The listing builds one solid part. Answer for the finished solid, in the listing's coordinates (mm). Give positions to 0.01 mm unless a question says otherwise; leave off trailing zeros. Write each loop counter-clockwise with the first axis right and the second up, starting at its lowest first coordinate (ties: lowest second). Pieces come first, ordered by that corner, then holes.
```python
from build123d import *
from build123d.topology import SkipClean

# Parameters (mm, degrees)
SKETCH1_R           = 31
SKETCH1_R_2         = 1.55
BOSS_EXTRUDE1_DEPTH = 2
BOSS_EXTRUDE2_START = 2
SKETCH3_R           = 11
BOSS_EXTRUDE2_DEPTH = 2
SKETCH4_R           = 4.5
CUT_EXTRUDE2_DEPTH  = 4
SKETCH2_R           = 8.2
CUT_EXTRUDE1_DEPTH  = 2


with BuildPart() as part:
    # Sketch1 → Boss-Extrude1 (new body)
    with BuildSketch(Plane.XY):
        Circle(SKETCH1_R)
        with Locations((-27, 0)):
            Circle(SKETCH1_R_2, mode=Mode.SUBTRACT)
        with Locations((-19.091883092, 19.091883092)):
            Circle(SKETCH1_R_2, mode=Mode.SUBTRACT)
        with Locations((0, 27)):
            Circle(SKETCH1_R_2, mode=Mode.SUBTRACT)
        with Locations((19.091883092, 19.091883092)):
            Circle(SKETCH1_R_2, mode=Mode.SUBTRACT)
        with Locations((27, 0)):
            Circle(SKETCH1_R_2, mode=Mode.SUBTRACT)
        with Locations((19.091883092, -19.091883092)):
            Circle(SKETCH1_R_2, mode=Mode.SUBTRACT)
        with Locations((0, -27)):
            Circle(SKETCH1_R_2, mode=Mode.SUBTRACT)
        with Locations((-19.091883092, -19.091883092)):
            Circle(SKETCH1_R_2, mode=Mode.SUBTRACT)
        with BuildLine():
            Line((-10.712142643, 2.5), (-22.86372673, 2.5))
            ThreePointArc((-22.86372673, 2.5), (-21.249229248, 8.801718944), (-17.934863167, 14.399329261))
            Line((-17.934863167, 14.399329261), (-9.342395657, 5.806861751))
            ThreePointArc((-9.342395657, 5.806861751), (-10.162674858, 4.209517756), (-10.712142643, 2.5))
        make_face(mode=Mode.SUBTRACT)
        with BuildLine():
            Line((-10.712142643, -2.5), (-22.86372673, -2.5))
            ThreePointArc((-22.86372673, -2.5), (-21.249229248, -8.801718944), (-17.934863167, -14.399329261))
            Line((-17.934863167, -14.399329261), (-9.342395657, -5.806861751))
            ThreePointArc((-9.342395657, -5.806861751), (-10.162674858, -4.209517756), (-10.712142643, -2.5))
        make_face(mode=Mode.SUBTRACT)
        with BuildLine():
            Line((-5.806861751, 9.342395657), (-14.399329261, 17.934863167))
            ThreePointArc((-14.399329261, 17.934863167), (-8.801718944, 21.249229248), (-2.5, 22.86372673))
            Line((-2.5, 22.86372673), (-2.5, 10.712142643))
            ThreePointArc((-2.5, 10.712142643), (-4.209517756, 10.162674858), (-5.806861751, 9.342395657))
        make_face(mode=Mode.SUBTRACT)
        with BuildLine():
            Line((2.5, 10.712142643), (2.5, 22.86372673))
            ThreePointArc((2.5, 22.86372673), (8.801718944, 21.249229248), (14.399329261, 17.934863167))
            Line((14.399329261, 17.934863167), (5.806861751, 9.342395657))
            ThreePointArc((5.806861751, 9.342395657), (4.209517756, 10.162674858), (2.5, 10.712142643))
        make_face(mode=Mode.SUBTRACT)
        with BuildLine():
            Line((9.342395657, 5.806861751), (17.934863167, 14.399329261))
            ThreePointArc((17.934863167, 14.399329261), (21.249229248, 8.801718944), (22.86372673, 2.5))
            Line((22.86372673, 2.5), (10.712142643, 2.5))
            ThreePointArc((10.712142643, 2.5), (10.162674858, 4.209517756), (9.342395657, 5.806861751))
        make_face(mode=Mode.SUBTRACT)
        with BuildLine():
            Line((10.712142643, -2.5), (22.86372673, -2.5))
            ThreePointArc((22.86372673, -2.5), (21.249229248, -8.801718944), (17.934863167, -14.399329261))
            Line((17.934863167, -14.399329261), (9.342395657, -5.806861751))
            ThreePointArc((9.342395657, -5.806861751), (10.162674858, -4.209517756), (10.712142643, -2.5))
        make_face(mode=Mode.SUBTRACT)
        with BuildLine():
            Line((5.806861751, -9.342395657), (14.399329261, -17.934863167))
            ThreePointArc((14.399329261, -17.934863167), (8.801718944, -21.249229248), (2.5, -22.86372673))
            Line((2.5, -22.86372673), (2.5, -10.712142643))
            ThreePointArc((2.5, -10.712142643), (4.209517756, -10.162674858), (5.806861751, -9.342395657))
        make_face(mode=Mode.SUBTRACT)
        with BuildLine():
            Line((-2.5, -10.712142643), (-2.5, -22.86372673))
            ThreePointArc((-2.5, -22.86372673), (-8.801718944, -21.249229248), (-14.399329261, -17.934863167))
            Line((-14.399329261, -17.934863167), (-5.806861751, -9.342395657))
            ThreePointArc((-5.806861751, -9.342395657), (-4.209517756, -10.162674858), (-2.5, -10.712142643))
        make_face(mode=Mode.SUBTRACT)
    extrude(amount=BOSS_EXTRUDE1_DEPTH)

    # Sketch3 → Boss-Extrude2 (add)
    with SkipClean():  # the faces are left unmerged after this step: merging them gives an invalid solid
        with BuildSketch(Plane(origin=(0, 0, 0), x_dir=(-1, 0, 0), z_dir=(0, 0, -1)).offset(BOSS_EXTRUDE2_START)):
            Circle(SKETCH3_R)
        extrude(amount=-BOSS_EXTRUDE2_DEPTH)

    # Sketch4 → Cut-Extrude2 (cut)
    with SkipClean():  # the faces are left unmerged after this step: merging them gives an invalid solid
        with BuildSketch(Plane.XY.offset(2)):
            Circle(SKETCH4_R)
        extrude(amount=-CUT_EXTRUDE2_DEPTH, mode=Mode.SUBTRACT)

    # Sketch2 → Cut-Extrude1 (cut)
    with SkipClean():  # the faces are left unmerged after this step: merging them gives an invalid solid
        with BuildSketch(Plane.XY.offset(2)):
            Circle(SKETCH2_R)
        extrude(amount=-CUT_EXTRUDE1_DEPTH, mode=Mode.SUBTRACT)


solid = part.part
```
Item 1: Each of these flat-tipped pins is pushed along its axis until it touches: P1, Ø3.5, axis at x = 19.09, y = -19.09, coming from the -Z side; P2, Ø1, axis at x = -16.5, z = 1.5, coming from the +Y side; P3, Ø2, axis at x = -15, z = 1, coming from the -Y side. Where does it stop, or does it pass through?
Conclusion:
P1: stops at z = 0
P2: stops at y = 26.55
P3: stops at y = -27.66
Item 2: Consider probe 1 along Y at (x, z) = (0, 0.05); probe 2 along Y at (x, z) = (-21, 1.7); probe 3 along Y at (x, z) = (5, 1.15). Determine where each line is inside the solid, lowest interval first.
Conclusion:
probe 1: y = -31 to -28.55, -25.45 to -8.2, 8.2 to 25.45, 28.55 to 31
probe 2: y = -22.8 to -9.38, -2.5 to 2.5, 9.38 to 22.8
probe 3: y = -30.59 to -22.45, -9.8 to -6.5, 6.5 to 9.8, 22.45 to 30.59
Item 3: Determine the mould class of faces 1 (the face through (18.89, 20.63, 0.99)), 2 (the face through (13, 0, 0)) for opening direction Y: pulls with the +Y half, pulls with the -Y half, needs draft (parallel to the pull), parting line crosses it, or undercut.
Conclusion:
face 1: undercut
face 2: needs draft
Item 4: A cutting plane is placed at A-A, the plane x = 0. Give the vertices of the cut face in (y, z), plus the area to 3 significant figures.
Conclusion:
outline: (-31, 0) - (-28.55, 0) - (-28.55, 2) - (-31, 2) - close; (-25.45, 0) - (-11, 0) - (-11, -2) - (-4.5, -2) - (-4.5, 0) - (-8.2, 0) - (-8.2, 2) - (-25.45, 2) - close; (4.5, -2) - (11, -2) - (11, 0) - (25.45, 0) - (25.45, 2) - (8.2, 2) - (8.2, 0) - (4.5, 0) - close; (28.55, 0) - (31, 0) - (31, 2) - (28.55, 2) - close
area: 105 mm2
Item 5: A cutting plane is placed at C-C, the plane x = -27. Give the vertices of the cut face in (y, z).
Conclusion:
outline: (-15.23, 0) - (-1.55, 0) - (-1.55, 2) - (-15.23, 2) - close; (1.55, 0) - (15.23, 0) - (15.23, 2) - (1.55, 2) - close
